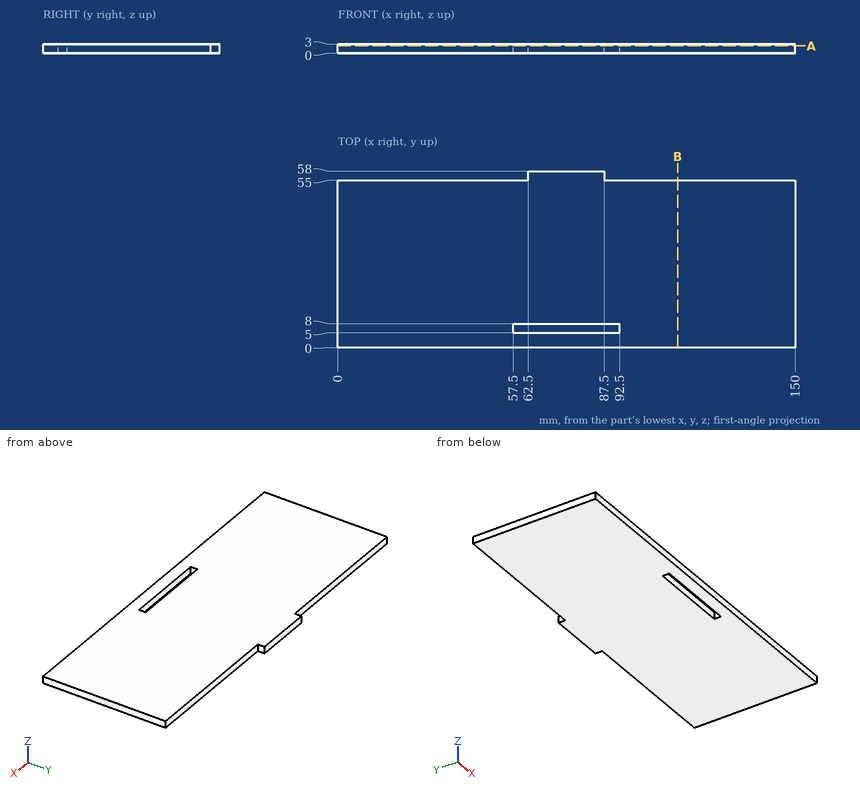
Input: dimensioned drawing with shaded views. Units: mm. Origin: part minimum x, y, z. Coordinates: 2 decimals unless noted, no trailing zeros. Loops run counter-clockwise (first coordinate to the right, second up) from the corner with the lowest first, then second, coordinate; pieces in that order, holes last. Notation, with made-up numbers: M 60,60 L 114,60 A18 ccw 114,88 Z; hole C 28.25,46 d8. An arc over 180 degrees is marked long. Use a Markdown table: item, result. Add a question column.
1) Line query: L1, parallel to Y at x = 61, z = 2.3; L2, parallel to Y at x = 87, z = 0.75; L3, parallel to Y at x = 113, z = 0.4. Output: solid intervals per line, ascending. Write a range as from..to.
2) Section A-A, the plane z = 2.35. Return the cut outline in (x, y), plus the area to 3 significant figures.
3) Section B-B, the plane x = 111.5. Return the cut outline in (y, z), plus the area to 3 significant figures.
4) Pin query (flat end, axial travel): P1, Ø1.5, axis at x = 30.5, z = 2, coming from the +Y side; P2, Ø0.9, axis at y = 57, z = 1.5, coming from the -X side. Return the tip coordinate at first contact, or that it passes through.
Answer below:
| question | item | result |
|---|---|---|
| 1 | L1 | 0..5, 8..55 |
| 1 | L2 | 0..5, 8..58 |
| 1 | L3 | 0..55 |
| 2 | outline | M 0,0 L 150,0 L 150,55 L 87.5,55 L 87.5,58 L 62.5,58 L 62.5,55 L 0,55 Z; hole M 57.5,5 L 92.5,5 L 92.5,8 L 57.5,8 Z |
| 2 | area | 8,220 mm2 |
| 3 | outline | M 0,0 L 55,0 L 55,3 L 0,3 Z |
| 3 | area | 165 mm2 |
| 4 | P1 | y = 55 |
| 4 | P2 | x = 62.5 |
